from build123d import *

# Parameters (mm, degrees)
SKETCH1_W           = 46
SKETCH1_H           = 27
BOSS_EXTRUDE1_DEPTH = 10
SKETCH2_W           = 60
SKETCH2_H           = 15
BOSS_EXTRUDE2_DEPTH = 20
SKETCH3_R           = 4
CUT_EXTRUDE2_DEPTH  = 65.420493634
SKETCH6_W           = 15
SKETCH6_H           = 5
BOSS_EXTRUDE4_DEPTH = 7
BOSS_EXTRUDE5_START = -21
BOSS_EXTRUDE5_DEPTH = 15
BOSS_EXTRUDE6_START = -21
BOSS_EXTRUDE6_DEPTH = 15
SKETCH12_W          = 15
SKETCH12_H          = 15
BOSS_EXTRUDE8_DEPTH = 40
SKETCH13_R          = 2.5
CUT_EXTRUDE4_DEPTH  = 40
FILLET1_START       = -21
FILLET1_DEPTH       = 15


with BuildPart() as part:
    # Sketch1 → Boss-Extrude1 (new body)
    with BuildSketch(Plane(origin=(0, 0, 0), x_dir=(1, 0, 0), z_dir=(0, 1, 0))):
        with Locations((23, 13.5)):
            Rectangle(SKETCH1_W, SKETCH1_H)
    extrude(amount=BOSS_EXTRUDE1_DEPTH)

    # Sketch2 → Boss-Extrude2 (add)
    with BuildSketch(Plane(origin=(0, 10, 0), x_dir=(1, 0, 0), z_dir=(0, 1, 0))):
        with Locations((23, 13.5)):
            Rectangle(SKETCH2_W, SKETCH2_H)
    extrude(amount=BOSS_EXTRUDE2_DEPTH)

    # Sketch3 → Cut-Extrude2 (cut, through all)
    with BuildSketch(Plane(origin=(0, 0, -21), x_dir=(-1, 0, 0), z_dir=(0, 0, -1))):
        with Locations((-44.5, 20)):
            Circle(SKETCH3_R)
        with Locations((-1.5, 20)):
            Circle(SKETCH3_R)
    extrude(amount=-CUT_EXTRUDE2_DEPTH, mode=Mode.SUBTRACT)

    # Sketch6 → Boss-Extrude4 (add)
    with BuildSketch(Plane.XY):
        with Locations((23, 7.5)):
            Rectangle(SKETCH6_W, SKETCH6_H)
    extrude(amount=BOSS_EXTRUDE4_DEPTH)

    # Boss-Extrude5: read off the stored shape, not the designer's step
    # Boss-Extrude5 outline → Boss-Extrude5 (add)
    with BuildSketch(Plane.XY.offset(BOSS_EXTRUDE5_START)):
        Polygon((-7, 10), (0, 0), (0, 10), align=None)
    extrude(amount=BOSS_EXTRUDE5_DEPTH)

    # Boss-Extrude6: read off the stored shape, not the designer's step
    # Boss-Extrude6 outline → Boss-Extrude6 (add)
    with BuildSketch(Plane.XY.offset(BOSS_EXTRUDE6_START)):
        Polygon((46, 0), (53, 10), (46, 10), align=None)
    extrude(amount=BOSS_EXTRUDE6_DEPTH)

    # Sketch12 → Boss-Extrude8 (add)
    with BuildSketch(Plane(origin=(0, 30, 0), x_dir=(1, 0, 0), z_dir=(0, 1, 0))):
        with Locations((38.5, 13.5)):
            Rectangle(SKETCH12_W, SKETCH12_H)
    extrude(amount=BOSS_EXTRUDE8_DEPTH)

    # Sketch13 → Cut-Extrude4 (cut)
    with BuildSketch(Plane(origin=(46, 0, 0), x_dir=(0, 0, -1), z_dir=(1, 0, 0))):
        with Locations((13.5, 60)):
            Circle(SKETCH13_R)
    extrude(amount=-CUT_EXTRUDE4_DEPTH, mode=Mode.SUBTRACT)

    # Fillet1: read off the stored shape, not the designer's step
    # Fillet1 outline → Fillet1 (add)
    with BuildSketch(Plane.XY.offset(FILLET1_START)):
        with BuildLine():
            Line((31, 30), (31, 50))
            add(Edge.make_bspline(
                [(31, 50), (31, 30), (21, 30)],
                knots=[0, 0, 0, 1, 1, 1], degree=2, weights=[1, 0.707106781, 1]))
            Line((21, 30), (31, 30))
        make_face()
        with BuildLine():
            add(Edge.make_bspline(
                [(46, 49.773719933), (46, 31.062015649), (53, 30)],
                knots=[0, 0, 0, 1, 1, 1], degree=2, weights=[1, 0.758287544, 1]))
            Line((46, 49.773719933), (46, 30))
            Line((46, 30), (53, 30))
        make_face()
    extrude(amount=FILLET1_DEPTH)


solid = part.part
Geometry check sheet. Reference: the model listing, model coordinates, mm. A direction names the side the tool comes from. Coordinates: 2 decimals unless noted, no trailing zeros. Loops run counter-clockwise (first coordinate to the right, second up) from the corner with the lowest first, then second, coordinate; pieces in that order, holes last. Notation, with made-up numbers: (32.5, 78) - (57.5, 78) arc R27 cw to (57.5, 97) - close; hole circle Ø1 at (8.25, 0.25). An arc over 180 degrees is marked (long way). Use one line per item in the form item = value. Start each with the question number.
Item 1: Thickness scan on probe 1 along Y at (x, z) = (1.5, -11); probe 2 along Z at (x, y) = (39, 35); probe 3 along Y at (x, z) = (42, -18). Record the ranges inside material, lowest first.
Item 2: Section check C-C, the plane y = 60. Enter the section's corners in (x, z).
Item 3: Section check B-B, the plane z = -13.5. Give the number of separate pieces and of enclosed holes in the cut face, and give its area (3 significant figures).
Item 4: Gauge pin test, flat ends, axial feed: pin 1 (1.5 mm diameter, centred on y = 7.5, z = 5, fed in from +X); pin 2 (14.5 mm diameter, centred on x = 32, z = 1.5, fed in from +Y); pin 3 (6 mm diameter, centred on x = 40, y = 46.5, fed in from -Z); pin 4 (7 mm diameter, centred on x = 1.5, y = 20, fed in from -Z). Record the tip position at first contact, or that the pin passes through.
Item 5: Mould release check, pull along Y, two halves, no side actions. Record for faces 4 (the face through (29, 28, -6)), 5 (the face through (39, 60, -11)), 6 (the face through (23, 5, 3)), 7 (the face through (2.021, 23.966, -13.605)): +Y half, -Y half, draft (parallel to the pull), parting line (faces both ways), or undercut.
Item 6: Tool access check on faces 1 (the face through (0, 5, -24)), 2 (the face through (31, 57.6, -15.1)), 3 (the face through (15.5, 7, 3)). Record the directions out of +Z, -Z, +X, -X, +Y, -Y that give a thin tool (end or side, any length) a straight path to the whole face; none if there is none.
Item 7: Section check D-D, the plane x = 1.5. Enter the section's corners in (y, z), and give its area (3 significant figures).
Item 8: Section check A-A, the plane x = 44.5. Enter the section's corners in (y, z).
Computed:
q1.probe_1 = 0 to 16, 24 to 30
q1.probe_2 = -21 to -6
q1.probe_3 = 0 to 16.88, 23.12 to 70
q2.outline = (31, -21) - (46, -21) - (46, -16) - (31, -16) - close; (31, -11) - (46, -11) - (46, -6) - (31, -6) - close
q3.separate_pieces = 2
q3.enclosed_holes = 2
q3.area = 2,230 mm2
q4.pin_1 = 30.5
q4.pin_2 = 10
q4.pin_3 = -21
q4.pin_4 = through
q5.face_4 = draft
q5.face_5 = undercut
q5.face_6 = -Y half
q5.face_7 = undercut
q6.face_1 = -Z, -X, +Y, -Y
q6.face_2 = +Z, -Z, -X, +Y
q6.face_3 = +Z, -X, +Y, -Y
q7.outline = (0, -27) - (10, -27) - (10, -21) - (16, -21) - (16, -6) - (10, -6) - (10, 0) - (0, 0) - close; (24, -21) - (30, -21) - (30, -6) - (24, -6) - close
q7.area = 450 mm2
q8.outline = (0, -27) - (10, -27) - (10, -21) - (16, -21) - (16, -6) - (10, -6) - (10, 0) - (0, 0) - close; (24, -21) - (70, -21) - (70, -6) - (24, -6) - close; hole circle Ø5 at (60, -13.5)
